from build123d import *

# Parameters (mm, degrees)
SKETCH_1_R      = 2.5
SKETCH_1_R_2    = 3
SKETCH_1_R_3    = 1.5
EXTRUDE_1_DEPTH = 3
FILLET_1_R      = 20
FILLET_2_R      = 5


with BuildPart() as part:
    # 草图1 → 凸台-拉伸1 (new body)
    with BuildSketch(Plane(origin=(0, 0, 0), x_dir=(1, 0, 0), z_dir=(0, 1, 0))):
        with BuildLine():
            Line((-35, -15), (-35, -45))
            ThreePointArc((-35, -45), (-34.121320344, -47.121320344), (-32, -48))
            Line((-32, -48), (32, -48))
            ThreePointArc((32, -48), (34.121320344, -47.121320344), (35, -45))
            Line((35, -45), (35, -15))
            Line((35, -15), (50, -15))
            Line((50, -15), (82.444008336, 4.297313883))
            ThreePointArc((82.444008336, 4.297313883), (88.512514494, 3.558404408), (89.330127019, -2.5))
            Line((89.330127019, -2.5), (74.509618943, -28.169872981))
            ThreePointArc((74.509618943, -28.169872981), (73.011112606, -31.787587305), (72.5, -35.669872981))
            Line((72.5, -35.669872981), (72.5, -67.5))
            Line((72.5, -67.5), (41.712797049, -67.5))
            Line((41.712797049, -67.5), (35, -75.5))
            Line((35, -75.5), (-35, -75.5))
            Line((-35, -75.5), (-41.712797049, -67.5))
            Line((-41.712797049, -67.5), (-72.5, -67.5))
            Line((-72.5, -67.5), (-72.5, -35.669872981))
            ThreePointArc((-72.5, -35.669872981), (-73.011112606, -31.787587305), (-74.509618943, -28.169872981))
            Line((-74.509618943, -28.169872981), (-89.330127019, -2.5))
            ThreePointArc((-89.330127019, -2.5), (-88.512514494, 3.558404408), (-82.444008336, 4.297313883))
            Line((-82.444008336, 4.297313883), (-50, -15))
            Line((-50, -15), (-35, -15))
        make_face()
        with Locations(Location((85, 0, 0), (0, 0, 270))):
            Circle(SKETCH_1_R, mode=Mode.SUBTRACT)
        with Locations(Location((-85, 0, 0), (0, 0, 270))):
            Circle(SKETCH_1_R, mode=Mode.SUBTRACT)
        with Locations(Location((47.5, -53, 0), (0, 0, 90))):
            Circle(SKETCH_1_R_2, mode=Mode.SUBTRACT)
        with Locations(Location((-47.5, -53, 0), (0, 0, 270))):
            Circle(SKETCH_1_R_2, mode=Mode.SUBTRACT)
        with Locations(Location((20, -55.5, 0), (0, 0, 270))):
            Circle(SKETCH_1_R_3, mode=Mode.SUBTRACT)
        with Locations(Location((-20, -55.5, 0), (0, 0, 270))):
            Circle(SKETCH_1_R_3, mode=Mode.SUBTRACT)
        with Locations(Location((-65, -55.5, 0), (0, 0, 270))):
            Circle(SKETCH_1_R_3, mode=Mode.SUBTRACT)
        with Locations(Location((65, -55.5, 0), (0, 0, 270))):
            Circle(SKETCH_1_R_3, mode=Mode.SUBTRACT)
        with Locations(Location((65, -20, 0), (0, 0, 270))):
            Circle(SKETCH_1_R_3, mode=Mode.SUBTRACT)
        with Locations(Location((-65, -20, 0), (0, 0, 270))):
            Circle(SKETCH_1_R_3, mode=Mode.SUBTRACT)
        with Locations(Location((40, -22.5, 0), (0, 0, 270))):
            Circle(SKETCH_1_R_3, mode=Mode.SUBTRACT)
        with Locations(Location((40, -30.5, 0), (0, 0, 270))):
            Circle(SKETCH_1_R_3, mode=Mode.SUBTRACT)
        with Locations(Location((-47.5, -27, 0), (0, 0, 270))):
            Circle(SKETCH_1_R_2, mode=Mode.SUBTRACT)
        with Locations(Location((47.5, -27, 0), (0, 0, 90))):
            Circle(SKETCH_1_R_2, mode=Mode.SUBTRACT)
        with Locations(Location((-40, -30.5, 0), (0, 0, 90))):
            Circle(SKETCH_1_R_3, mode=Mode.SUBTRACT)
        with Locations(Location((-40, -22.5, 0), (0, 0, 90))):
            Circle(SKETCH_1_R_3, mode=Mode.SUBTRACT)
    extrude(amount=EXTRUDE_1_DEPTH)

    # 圆角1
    fillet_1_edges = [part.edges().sort_by_distance(p)[0] for p in [
        (50, 1.5, 15),
        (-50, 1.5, 15),
    ]]
    fillet(fillet_1_edges, radius=FILLET_1_R)

    # 圆角2
    fillet_2_edges = [part.edges().sort_by_distance(p)[0] for p in [
        (35, 1.5, 15),
        (72.5, 1.5, 67.5),
        (41.712797049, 1.5, 67.5),
        (35, 1.5, 75.5),
        (-35, 1.5, 75.5),
        (-41.712797049, 1.5, 67.5),
        (-72.5, 1.5, 67.5),
        (-35, 1.5, 15),
    ]]
    fillet(fillet_2_edges, radius=FILLET_2_R)


solid = part.part
Design review of the part built by this model. Coordinates are the model's own, in mm. A direction names the side the tool comes from. Round coordinates to 2 decimals unless told otherwise and drop trailing zeros. Order: outer loops, then holes, each group sorted by start corner. A loop starts at its lowest first (then second) coordinate and runs counter-clockwise, first axis right, second up. Notation, with made-up numbers: M 44,32 L 62,32 A22 ccw 62,38 Z; hole C 89.25,86.5 d4. An arc over 180 degrees is marked long. Answer as CSV lines item,"result". Start each with the question number.
1) For pin 1 Ø1.5 at (x, y) = (42, 2) entering from -Z; pin 2 Ø1.5 at (y, z) = (0.5, 31.5) entering from +X; pin 3 Ø0.9 at (y, z) = (2, 37) entering from +X, all flat-tipped, find the tip position at first contact; note any pin that passes through.
2) Add section A-A (x = 85). Give the boundary of the cut face in (y, z).
3) Add section B-B (z = 10.5). Give the boundary of the cut face in (x, y), then the cut area to 3 significant figures.
4) Wall thickness on line 1 along X through (y, z) = (1.85, 53); line 2 along X through (y, z) = (1.2, 20); line 3 along X through (y, z) = (2.4, 0): over which ranges is each line inside the solid? List them lowest first. Write a range as [from, to].
5) The part is to be moulded in two halves that separate along Z. For faces 4 (the face through (-42, 1, 15)), 5 (the face through (-89, 1, -3)), 6 (the face through (87.48, 1.48, -0.33)), 7 (the face through (-82.52, 1.48, -0.33)), say which applies: +Z half, -Z half, draft (parallel to the pull), parting line (faces both ways), or undercut.
6) Add section C-C (y = 2.3). Give the number of separate pieces and of enclosed holes in the cut face, then the cut area to 3 significant figures.
7) Tool access review of faces 1 (the face through (-49.731, 1.521, 14.304)), 2 (the face through (56, 1, 67.5)), 3 (the face through (-72.5, 1, 49)): name each direction out of +Z, -Z, +X, -X, +Y, -Y from which nothing blocks a thin tool from reaching the whole face with its end or side.
Resolved:
1,pin 1,"z = 15"
1,pin 2,"x = 73.33"
1,pin 3,"x = 72.5"
2,outline,"M 0,-5 L 3,-5 L 3,-2.5 L 0,-2.5 Z; M 0,2.5 L 3,2.5 L 3,10 L 0,10 Z"
3,outline,"M -84.71,0 L -57.57,0 L -57.57,3 L -84.71,3 Z; M 57.57,0 L 84.71,0 L 84.71,3 L 57.57,3 Z"
3,area,"163 mm^2"
4,line 1,"[-72.5, -50.5], [-44.5, 44.5], [50.5, 72.5]"
4,line 2,"[-79.23, -66.5], [-63.5, -35], [35, 63.5], [66.5, 79.23]"
4,line 3,"[-90, -87.5], [-82.5, -75.22], [75.22, 82.5], [87.5, 90]"
5,face 4,"-Z half"
5,face 5,"parting line"
5,face 6,"undercut"
5,face 7,"undercut"
6,separate pieces,"1"
6,enclosed holes,"16"
6,area,"6,650 mm^2"
7,face 1,"-Z, +Y, -Y"
7,face 2,"+Z, +X, +Y, -Y"
7,face 3,"+Z, -X, +Y, -Y"
